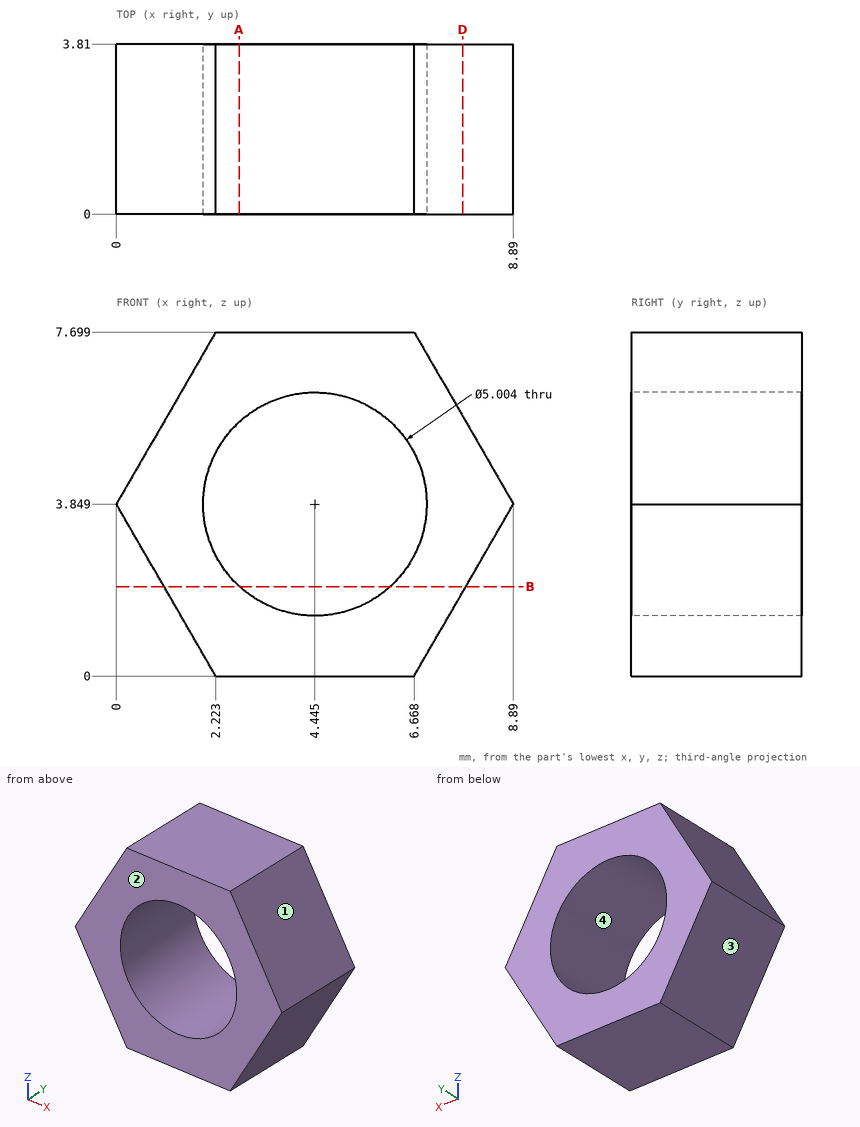
Geometry check sheet. Reference: drawing and pictorial views, mm from the part's lowest x, y, z. Coordinates: 2 decimals unless noted, no trailing zeros. Order: outer loops, then holes, each group sorted by start corner. A loop starts at its lowest first (then second) coordinate and runs counter-clockwise, first axis right, second up. Notation, with made-up numbers: (81.5, 15) -> (122.5, 15) arc R12 ccw to (122.5, 36) -> close; hole circle Ø3 at (9, 35.5). An arc over 180 degrees is marked (long way). Use CSV: the item, a comma, the result in double quotes. Start each with the question number.
Q1. Thickness scan on line 1 along Z through (x, y) = (4.5, 0.7); line 2 along Z through (x, y) = (3.75, 3.25) (1 decimal); line 3 along X through (y, z) = (3.55, 2) (1 decimal). Record the ranges inside material, lowest first.
Q2. Draft check along X on the marked faces 1, 2, 3 and 4. Enter one of: +X half, -X half, draft (parallel to the pull), parting line (faces both ways), or undercut.
Q3. Section check B-B, the plane z = 2. Record the cut outline in (x, y), and give its area (3 significant figures).
Q4. Section check D-D, the plane x = 7.75. Record the cut outline in (y, z) (1 decimal).
Q5. Section check A-A, the plane x = 2.75. Record the cut outline in (y, z).
Q6. Depth check by flat-ended pin: P1, Ø1.5, axis at x = 1, y = 1.5, coming from the -Z side; P2, Ø1, axis at y = 2.5, z = 5, coming from the +X side (1 decimal); P3, Ø1.5, axis at x = 4, z = 4, coming from the +Y side. Enter the tip coordinate at first touch or a pass-through.
Returned:
1,line 1,"z = 0 to 1.35, 6.35 to 7.7"
1,line 2,"z = 0 to 1.4, 6.3 to 7.7"
1,line 3,"x = 1.1 to 2.8, 6.1 to 7.8"
2,face 1,"+X half"
2,face 2,"draft"
2,face 3,"-X half"
2,face 4,"undercut"
3,outline,"(1.07, 0) -> (2.76, 0) -> (2.76, 3.81) -> (1.07, 3.81) -> close; (6.13, 0) -> (7.82, 0) -> (7.82, 3.81) -> (6.13, 3.81) -> close"
3,area,"12.9 mm^2"
4,outline,"(0, 1.9) -> (3.8, 1.9) -> (3.8, 5.8) -> (0, 5.8) -> close"
5,outline,"(0, 0) -> (3.81, 0) -> (3.81, 2.01) -> (0, 2.01) -> close; (0, 5.69) -> (3.81, 5.69) -> (3.81, 7.7) -> (0, 7.7) -> close"
6,P1,"stops at z = 0.82"
6,P2,"stops at x = 8.5"
6,P3,"passes through"
